Could you check a few things on this drawing? It's one solid part, dimensions in mm from its lowest x, y, z. Coordinates: 2 decimals unless noted, no trailing zeros. Write each loop counter-clockwise with the first axis right and the second up, starting at its lowest first coordinate (ties: lowest second). Pieces come first, ordered by that corner, then holes.
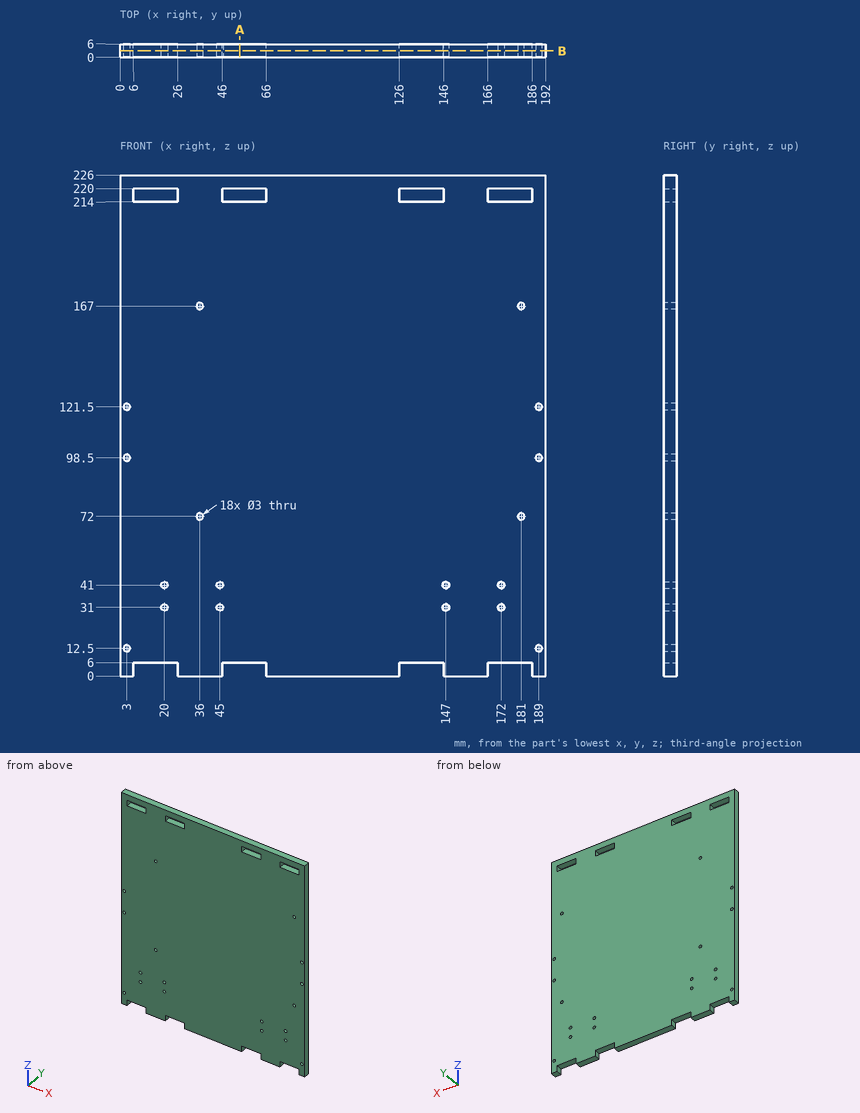
1) I need wall thicknesses on probe 1 along Z at (x, y) = (20, 2.45); probe 2 along X at (y, z) = (4.45, 167); probe 3 along X at (y, z) = (2.9, 31). Which ranges of each line are inside material? Lowest first, please.
Values follow:
probe 1: z = 6 to 29.5, 32.5 to 39.5, 42.5 to 214, 220 to 226
probe 2: x = 0 to 34.5, 37.5 to 179.5, 182.5 to 192
probe 3: x = 0 to 18.5, 21.5 to 43.5, 46.5 to 145.5, 148.5 to 170.5, 173.5 to 192
2) Imagine slicing it at A-A on x = 54. Please give me the cut outline in (y, z), then the cut area to 3 significant figures.
Values follow:
outline: (0, 6) - (6, 6) - (6, 214) - (0, 214) - close; (0, 220) - (6, 220) - (6, 226) - (0, 226) - close
area: 1,280 mm2
3) Imagine slicing it at B-B on y = 2.9. Count the separate pieces of the cut face and the enclosed holes in it, then the cut area to 3 significant figures.
Values follow:
separate pieces: 1
enclosed holes: 22
area: 42,300 mm2
4) Will this pin go through, and if not, where does the flat tip stop? pin 1 (1.8 mm diameter, centred on x = 179, y = 2, fed in from -Z).
Values follow:
pin 1: stops at z = 6
